Verification items for the finished model (mm, model axes). A direction names the side the tool comes from. Round coordinates to 2 decimals unless told otherwise and drop trailing zeros. Write each loop counter-clockwise with the first axis right and the second up, starting at its lowest first coordinate (ties: lowest second). Pieces come first, ordered by that corner, then holes. Notation, with made-up numbers: (83.5, -22.5) - (137.5, -22.5) arc R29 ccw to (137.5, 1.5) - close; hole circle Ø8 at (-2.75, -27). An arc over 180 degrees is marked (long way). Write each question's results on one line, items separated by ' | '.
```python
from build123d import *

# Parameters (mm, degrees)
BASE_FLANGE1_DEPTH = 10
SKETCH6_R          = 2.55
CUT_EXTRUDE1_DEPTH = 21.14944168


# Sheet-metal steps are written as plain solids
with BuildPart() as part:
    # Sketch1 → Base-Flange1 (new body)
    with BuildSketch(Plane.XY):
        with BuildLine():
            Line((0, 15), (0, 0.7366))
            ThreePointArc((0, 0.7366), (0.215745145, 0.215745145), (0.7366, 0))
            Line((0.7366, 0), (4.2634, 0))
            ThreePointArc((4.2634, 0), (4.784254855, 0.215745145), (5, 0.7366))
            Line((5, 0.7366), (5, 15))
            Line((5, 15), (7, 15))
            Line((7, 15), (7, 0.7366))
            ThreePointArc((7, 0.7366), (6.198468417, -1.198468417), (4.2634, -2))
            Line((4.2634, -2), (0.7366, -2))
            ThreePointArc((0.7366, -2), (-1.198468417, -1.198468417), (-2, 0.7366))
            Line((-2, 0.7366), (-2, 15))
            Line((-2, 15), (0, 15))
        make_face()
    extrude(amount=BASE_FLANGE1_DEPTH)

    # Sketch6 → Cut-Extrude1 (cut, through all)
    with BuildSketch(Plane.ZY.offset(2)):
        with Locations((5, 10)):
            Circle(SKETCH6_R)
    extrude(amount=-CUT_EXTRUDE1_DEPTH, mode=Mode.SUBTRACT)


solid = part.part
```
(1) Section check C-C (y = 10). Record the cut outline in (x, z), plus the area to 3 significant figures.
Answer:
outline: (-2, 0) - (0, 0) - (0, 2.45) - (-2, 2.45) - close; (-2, 7.55) - (0, 7.55) - (0, 10) - (-2, 10) - close; (5, 0) - (7, 0) - (7, 2.45) - (5, 2.45) - close; (5, 7.55) - (7, 7.55) - (7, 10) - (5, 10) - close | area: 19.6 mm2
(2) Go/stop test with flat-tipped pins: pin 1 Ø3 at (x, z) = (2.5, 7.5) entering from +Y; pin 2 Ø4.5 at (y, z) = (10, 5) entering from +X. Record where each tip stops, or that it passes through.
Answer:
pin 1: y = 0 | pin 2: through
(3) Section check B-B (y = 2.75). Record the cut outline in (x, z).
Answer:
outline: (-2, 0) - (0, 0) - (0, 10) - (-2, 10) - close; (5, 0) - (7, 0) - (7, 10) - (5, 10) - close
(4) Mould release check, pull along Z, two halves, no side actions. Record for faces 3 (the flat face through (2, 0, 5)), 4 (the cylindrical face through (5.99, 7.74, 6.18)), 5 (the cylindrical face through (-1.01, 7.74, 6.18)), 6 (the flat face through (6, 7, 0)): released by +Z, released by -Z, zero draft, split by the parting line, or undercut.
Answer:
face 3: zero draft | face 4: undercut | face 5: undercut | face 6: released by -Z
(5) Set-up check for faces 1 (the flat face through (5, 6, 5)), 2 (the flat face through (6, 7, 10)): record each of +Z, -Z, +X, -X, +Y, -Y from which the full face is reachable in a straight line by a thin tool's end or side.
Answer:
face 1: +Z, -Z, +Y | face 2: +Z, +X, -X, +Y, -Y
(6) Thickness scan on L1, parallel to X at y = 13.75, z = 2.25; L2, parallel to Y at x = 4, z = 6; L3, parallel to Y at x = -1.5, z = 5. Record the ranges inside material, lowest first.
Answer:
L1: -2 to 0, 5 to 7 | L2: -2 to 0 | L3: -0.84 to 7.45, 12.55 to 15
(7) Section check D-D (z = 1.5). Record the cut outline in (x, y), plus the area to 3 significant figures.
Answer:
outline: (-2, 0.74) arc R2.74 ccw to (0.74, -2) - (4.26, -2) arc R2.74 ccw to (7, 0.74) - (7, 15) - (5, 15) - (5, 0.74) arc R0.74 cw to (4.26, 0) - (0.74, 0) arc R0.74 cw to (0, 0.74) - (0, 15) - (-2, 15) - close | area: 75.0 mm2
(8) Section check A-A (z = 5). Record the cut outline in (x, y).
Answer:
outline: (-2, 0.74) arc R2.74 ccw to (0.74, -2) - (4.26, -2) arc R2.74 ccw to (7, 0.74) - (7, 7.45) - (5, 7.45) - (5, 0.74) arc R0.74 cw to (4.26, 0) - (0.74, 0) arc R0.74 cw to (0, 0.74) - (0, 7.45) - (-2, 7.45) - close; (-2, 12.55) - (0, 12.55) - (0, 15) - (-2, 15) - close; (5, 12.55) - (7, 12.55) - (7, 15) - (5, 15) - close
